from build123d import *

# Parameters (mm, degrees)
PAD009_DEPTH    = 2.8
FILLET004_R     = 0.4
POCKET014_DEPTH = 2.801


with BuildPart() as part:
    # Sketch009 → Pad009 (new body)
    with BuildSketch(Plane.XZ.offset(60.5)):
        with BuildLine():
            Line((37.8, 3.2), (37.8, 0.4))
            Line((37.8, 0.4), (23.8, 0.4))
            ThreePointArc((23.8, 0.4), (23.4, 0), (23.8, -0.4))
            Line((23.8, -0.4), (37.8, -0.4))
            Line((37.8, -0.4), (37.8, -33.8))
            Line((37.8, -33.8), (23.8, -33.8))
            ThreePointArc((23.8, -33.8), (23.4, -34.2), (23.8, -34.6))
            Line((23.8, -34.6), (37.8, -34.6))
            Line((37.8, -34.6), (37.8, -37.4))
            Line((37.8, -37.4), (35.8, -38.4))
            Line((35.8, -38.4), (35.8, -37.4))
            Line((35.8, -37.4), (33, -37.4))
            Line((33, -37.4), (33, -39.4))
            Line((33, -39.4), (25.535898, -37.4))
            Line((25.535898, -37.4), (-25.535898, -37.4))
            Line((-25.535898, -37.4), (-33, -39.4))
            Line((-33, -39.4), (-33, -37.4))
            Line((-33, -37.4), (-35.8, -37.4))
            Line((-35.8, -38.4), (-35.8, -37.4))
            Line((-37.8, -37.4), (-35.8, -38.4))
            Line((-37.8, -37.4), (-37.8, -34.6))
            Line((-37.8, -34.6), (-23.8, -34.6))
            ThreePointArc((-23.8, -34.6), (-23.4, -34.2), (-23.8, -33.8))
            Line((-23.8, -33.8), (-37.8, -33.8))
            Line((-37.8, -33.8), (-37.8, -0.4))
            Line((-37.8, -0.4), (-23.8, -0.4))
            ThreePointArc((-23.8, -0.4), (-23.4, 0), (-23.8, 0.4))
            Line((-23.8, 0.4), (-37.8, 0.4))
            Line((-37.8, 0.4), (-37.8, 3.2))
            Line((-37.8, 3.2), (-35.8, 4.2))
            Line((-35.8, 4.2), (-35.8, 3.2))
            Line((-35.8, 3.2), (-33, 3.2))
            Line((-33, 3.2), (-33, 5.2))
            Line((-33, 5.2), (-25.535898, 3.2))
            Line((-25.535898, 3.2), (25.535898, 3.2))
            Line((25.535898, 3.2), (33, 5.2))
            Line((33, 5.2), (33, 3.2))
            Line((33, 3.2), (35.8, 3.2))
            Line((35.8, 3.2), (35.8, 4.2))
            Line((37.8, 3.2), (35.8, 4.2))
        make_face()
    extrude(amount=-PAD009_DEPTH)

    # Fillet004
    fillet004_edges = [part.edges().sort_by_distance(p)[0] for p in [
        (37.8, -59.1, -0.4),
        (37.8, -59.1, 0.4),
        (37.8, -59.1, 3.2),
        (25.535898, -59.1, 3.2),
        (-25.535898, -59.1, 3.2),
        (-37.8, -59.1, 3.2),
        (-37.8, -59.1, 0.4),
        (-37.8, -59.1, -0.4),
        (-37.8, -59.1, -33.8),
        (-37.8, -59.1, -34.6),
        (-37.8, -59.1, -37.4),
        (-25.535898, -59.1, -37.4),
        (25.535898, -59.1, -37.4),
        (37.8, -59.1, -37.4),
        (37.8, -59.1, -34.6),
        (37.8, -59.1, -33.8),
    ]]
    fillet(fillet004_edges, radius=FILLET004_R)

    # Sketch025 → Pocket014 (cut, through all)
    with BuildSketch(Plane.XZ.offset(60.5)):
        with BuildLine():
            ThreePointArc((-24, -4.49), (-24.755, -5.245), (-24, -6))
            Line((-24, -6), (-12, -6))
            ThreePointArc((-12, -6), (-11.245, -5.245), (-12, -4.49))
            Line((-24, -4.49), (-12, -4.49))
        make_face()
        with BuildLine():
            ThreePointArc((12, -4.49), (11.245, -5.245), (12, -6))
            Line((12, -6), (24, -6))
            ThreePointArc((24, -6), (24.755, -5.245), (24, -4.49))
            Line((12, -4.49), (24, -4.49))
        make_face()
    extrude(amount=-POCKET014_DEPTH, mode=Mode.SUBTRACT)


solid = part.part
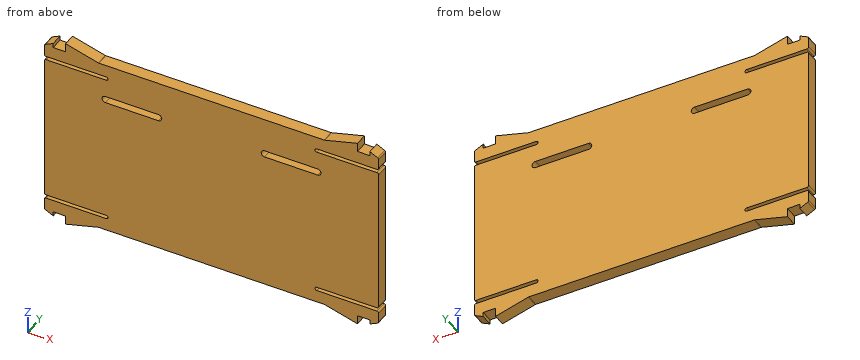
Geometry check sheet. Reference: the model listing, model coordinates, mm. Give positions to 0.01 mm unless a question says otherwise; leave off trailing zeros. Write each loop counter-clockwise with the first axis right and the second up, starting at its lowest first coordinate (ties: lowest second). Pieces come first, ordered by that corner, then holes. Notation, with made-up numbers: M 35.5,27 L 86.5,27 A16 cw 86.5,55 Z; hole C -33,1.5 d8. An arc over 180 degrees is marked long. Answer as CSV lines item,"result". Start each with the question number.
Q1. Section check B-B, the plane x = 27. Record the cut outline in (y, z).
Q2. Go/stop test with flat-tipped pins: pin 1 (1 mm diameter, centred on y = -59, z = 4, fed in from -X); pin 2 (1.4 mm diameter, centred on x = 12.5, y = -59.5, fed in from +Z); pin 3 (1.4 mm diameter, centred on x = 28.5, y = -59, fed in from -Z). Record where each tip stops, or that it passes through.
Q3. Section check A-A, the plane x = -15. Record the cut outline in (y, z), then the cut area to 3 significant figures.
Q4. Material ranges on L1, parallel to Z at x = 24, y = -58.05; L2, parallel to Z at x = 34.5, y = -59.45; L3, parallel to Z at x = -17.5, y = -58.9, recorded low to high.
Q5. Section check C-C, the plane y = -59.6. Give the number of separate pieces and of enclosed holes in the cut face, then the cut area to 3 significant figures.
Geometry says:
1,outline,"M -60.5,-37.79 L -57.7,-37.79 L -57.7,-34.6 L -60.5,-34.6 Z; M -60.5,-33.8 L -57.7,-33.8 L -57.7,-0.4 L -60.5,-0.4 Z; M -60.5,0.4 L -57.7,0.4 L -57.7,3.59 L -60.5,3.59 Z"
2,pin 1,"x = -37.2"
2,pin 2,"z = 3.2"
2,pin 3,"z = -38.38"
3,outline,"M -60.5,-37.4 L -57.7,-37.4 L -57.7,-6 L -60.5,-6 Z; M -60.5,-4.49 L -57.7,-4.49 L -57.7,3.2 L -60.5,3.2 Z"
3,area,"109 mm^2"
4,L1,"-37.4 to -34.6, -33.8 to -6, -4.49 to -0.4, 0.4 to 3.2"
4,L2,"-37.4 to -34.6, -33.8 to -0.4, 0.4 to 3.2"
4,L3,"-37.4 to -6, -4.49 to 3.2"
5,separate pieces,"1"
5,enclosed holes,"2"
5,area,"3,020 mm^2"
